Here's how the part is built. I have some questions about the finished solid (model axes, mm). A direction names the side the tool comes from. Coordinates: 2 decimals unless noted, no trailing zeros. Loops run counter-clockwise (first coordinate to the right, second up) from the corner with the lowest first, then second, coordinate; pieces in that order, holes last. Notation, with made-up numbers: (67, 60) -> (71, 60) arc R13 cw to (71, 79) -> close; hole circle Ø9 at (50, 61). An arc over 180 degrees is marked (long way). Answer as a JSON object with one key per item and string values. Group by question number.
Q1. I want a section at C-C on y = 6. Write out the boundary of the cut face in (x, z), then the cut area to 3 significant figures.
Q2. I want a section at B-B on x = -1.5. Count the separate pieces of the cut face and the enclosed holes in it, then the cut area to 3 significant figures.
Q3. On a 3-axis mill with a long thin cutter (end or side, diameter ignored), from which of +Z, -Z, +X, -X, +Y, -Y can I reach the whole of each face in a straight line? I mean faces 1 (the flat face through (0, 0, 0)), 2 (the cylindrical face through (-2.8, 21.8, 14.6)), 3 (the cylindrical face through (-0.108, 33.142, 12.544)). Say none if no direction works.
Q4. I need wall thicknesses on line 1 (Z direction, x = 0, y = 35); line 2 (X direction, y = 30, z = -15); line 3 (Z direction, x = 0.5, y = 20). Which ranges of each line are inside material? Lowest first, please.
Q5. I want a section at A-A on y = 32. Write out the boundary of the cut face in (x, z).
Q6. I'm going to push flat-ended pins straight in: pin 1 (5 mm diameter, centred on y = 20, z = 17, fed in from -X); pin 2 (5.5 mm diameter, centred on x = 0, z = 15, fed in from +Y); pin 3 (6 mm diameter, centred on y = 20, z = 0, fed in from -X). Where does each tip first touch, or does it pass through?
Q7. Thinking about a two-plate mould opening in Z: for faces 4 (the cylindrical face through (-2.8, 21.8, -19.4)), 5 (the flat face through (9.507, 10.14, 0.35)), 6 (the flat face through (0, 20, 25)), 7 (the conical face through (0.02, 25.78, 14.57)), which applies, released by +Z, released by -Z, zero draft, split by the parting line, or undercut?
Autodesk Inventor part; units mm, degrees
ref_plane "YZ Plane" through (0, 0, 0) normal (1, 0, 0) x (0, 1, 0)
ref_plane "XZ Plane" through (0, 0, 0) normal (0, 1, 0) x (-1, 0, 0)
ref_plane "XY Plane" through (0, 0, 0) normal (0, 0, 1) x (1, 0, 0)
sketch "Sketch2" plane through (0, 0, 0) normal (0, 1, 0) x (-1, 0, 0)
  line L0 (-10, 25) -> (10, 25)
  line L1 (10, 25) -> (10, -25)
  line L2 (10, -25) -> (-10, -25)
  line L3 (-10, -25) -> (-10, 25)
  line L4 (-10, 25) -> (10, -25) construction
  line L5 (10, 25) -> (-10, -25) construction
  point P0 (0, 0)
  dimension "d0" = 50
  dimension "d1" = 20
extrude "Extrusion1" add sketch "Sketch2" along normal blind 40
sketch "Sketch3" plane through (-10, 0, 25) normal (0, 0, 1) x (1, 0, 0)
  line L0 (20, 0) -> (20, 40)
  line L1 (20, 40) -> (20, 20)
  line L2 (0, 40) -> (20, 40)
  line L3 (20, 20) -> (19, 0)
  line L4 (20, 0) -> (0, 0)
  line L5 (19, 0) -> (20, 0)
  line L6 (20, 0) -> (20, 20)
  point P0 (10, 0)
  dimension "d4" = 20
  dimension "d5" = 1
extrude "Extrusion2" cut sketch "Sketch3" against normal through all
sketch "Sketch4" plane through (-10, 0, -25) normal (-1, 0, 0) x (0, 0, 1)
  line L0 (0, 0) -> (0, 40)
  line L1 (50, 0) -> (50, 40)
  line L2 (25, 0) -> (25, 40) construction
  line L3 (50, 40) -> (0, 40)
  line L4 (0, 20) -> (50, 20) construction
  line L5 (0, 0) -> (50, 0)
  point P0 (8, 20)
  point P1 (42, 20)
  point P2 (25, 20)
  dimension "d8" = 8
  dimension "d9" = 8
  dimension "d10" = 20
hole "Hole1" at (-10, 20, -17) at (-10, 20, 17) direction (1, 0, 0) diameter 6 depth 14 tip angle 118 countersink diameter 6.2 countersink angle 45
hole "Hole2" at (-10, 20, 0) direction (1, 0, 0) diameter 6.647 depth 14 tip angle 118 countersink diameter 8 countersink angle 45
sketch "Sketch5" plane through (0, 40, 0) normal (0, 1, 0) x (1, 0, 0)
  line L0 (10, 25) -> (-10, 25)
  line L1 (-10, 25) -> (-10, -25)
  line L2 (-10, -25) -> (10, -25)
  line L3 (10, -25) -> (10, 25)
  line L4 (0, 25) -> (0, -25) construction
  point P0 (0, 0)
  point P1 (0, 15)
  point P2 (0, -15)
  point P3 (0, 0)
  dimension "d25" = 15
  dimension "d26" = 15
hole "Hole3" at (0, 40, -15) at (0, 40, 15) direction (0, -1, 0) diameter 4.917 depth 13 tip angle 118 countersink diameter 6 countersink angle 90
equation "\"d0\" = Länge_Backe"
equation "\"d1\" = Breite_Backe"
equation "\"d2\" = Höhe_Backe"
equation "\"d4\" = Absatz_Höhe"
equation "\"d5\" = 0.5 * Max_Versatz"
equation "\"d10\" = Höhe_Schrauben"
equation "\"d11\" = Bolzen_Durchmesser"
equation "\"Breite_Backe\" = 20"
equation "\"Höhe_Backe\" = 40"
equation "\"Länge_Backe\" = 50"
equation "\"Absatz_Höhe\" = 20"
equation "\"Max_Versatz\" = 2"
equation "\"Abstand_Bolzen\" = 8"
equation "\"Höhe_Schrauben\" = 20"
equation "\"Bolzen_Durchmesser\" = 6"
properties part number "ER_Positionierungseinheit_Backe_int"
Result set:
{
 "1": {"outline": "(-10, -25) -> (9.3, -25) -> (9.3, 25) -> (-10, 25) -> close", "area": "965 mm²"},
 "2": {"separate pieces": "1", "enclosed holes": "3", "area": "1,800 mm²"},
 "3": {"face 1": "+Z, -Z, +X, -X, -Y", "face 2": "-X", "face 3": "+Y"},
 "4": {"line 1": "z = -25 to -17.46, -12.54 to 12.54, 17.46 to 25", "line 2": "x = -10 to -2.46, 2.46 to 10", "line 3": "z = -25 to -20, -14 to -3.32, 3.32 to 14, 20 to 25"},
 "5": {"outline": "(-10, -25) -> (10, -25) -> (10, 25) -> (-10, 25) -> close; hole circle Ø4.92 at (0, -15); hole circle Ø4.92 at (0, 15)"},
 "6": {"pin 1": "stops at x = 4.3", "pin 2": "stops at y = 39.75", "pin 3": "stops at x = 4.19"},
 "7": {"face 4": "undercut", "face 5": "zero draft", "face 6": "released by +Z", "face 7": "undercut"}
}
